Source: three-view drawing plus pictorial views. Frame: mm from the lowest corner of the part. Give positions to 0.01 mm unless a question says otherwise; leave off trailing zeros. Loops run counter-clockwise (first coordinate to the right, second up) from the corner with the lowest first, then second, coordinate; pieces in that order, holes last.
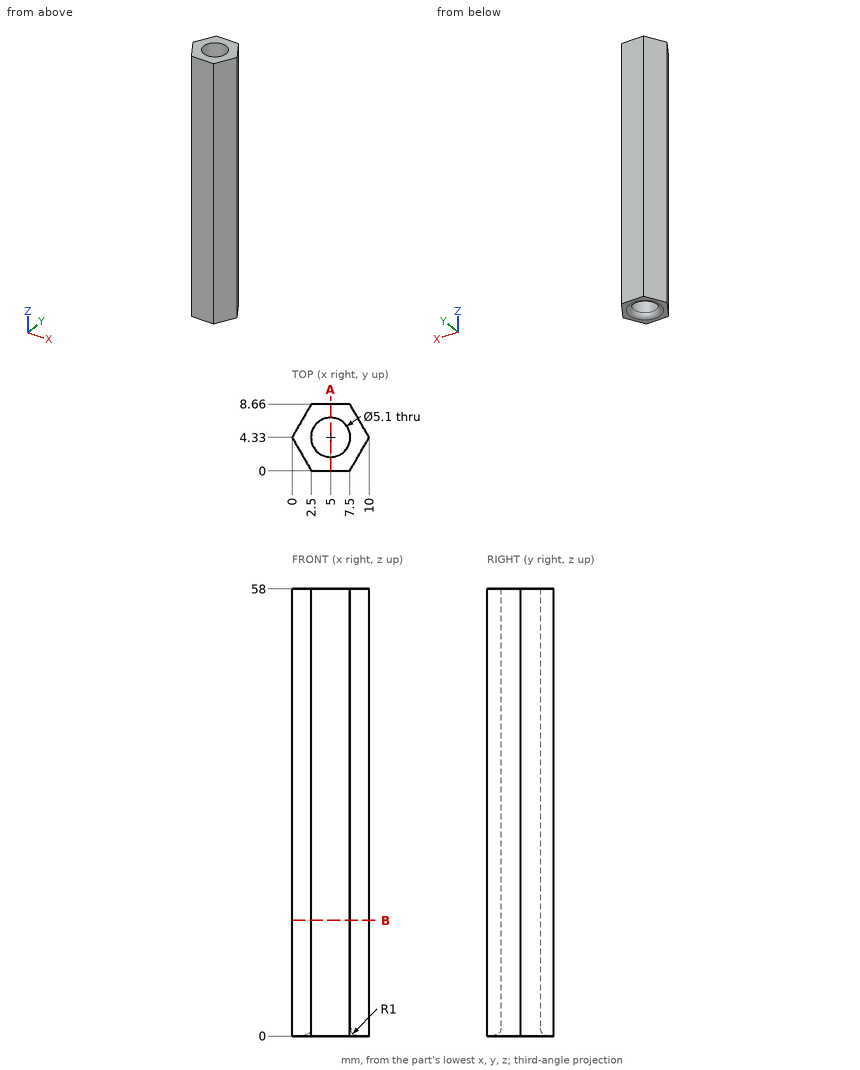
(1) Cut plane A-A (x = 5). Return the cut outline in (y, z), and give its area (3 significant figures).
Values follow:
outline: (0, 0) - (0.78, 0) arc R1 ccw to (1.78, 1) - (1.78, 58) - (0, 58) - close; (6.88, 1) arc R1 ccw to (7.88, 0) - (8.66, 0) - (8.66, 58) - (6.88, 58) - close
area: 206 mm2
(2) Cut plane B-B (z = 15). Return the cut outline in (x, y), and give its area (3 significant figures).
Values follow:
outline: (0, 4.33) - (2.5, 0) - (7.5, 0) - (10, 4.33) - (7.5, 8.66) - (2.5, 8.66) - close; hole circle Ø5.1 at (5, 4.33)
area: 44.5 mm2
(3) Ray query, probe 1 along Y at (x, z) = (5, 16); probe 2 along Y at (x, z) = (4.5, 25); probe 3 along X at (y, z) = (3.75, 52.5) (1 decimal). Return the intervals inside material, ascending.
Values follow:
probe 1: y = 0 to 1.78, 6.88 to 8.66
probe 2: y = 0 to 1.83, 6.83 to 8.66
probe 3: x = 0.3 to 2.5, 7.5 to 9.7
